Source: CAD feature listing. Evaluate the final solid. Frame: model axes, mm. Face numbers are marked on the shaded views. A direction names the side the tool comes from. Give positions to 0.01 mm unless a question says otherwise; leave off trailing zeros. Write each loop counter-clockwise with the first axis right and the second up, starting at its lowest first coordinate (ties: lowest second). Pieces come first, ordered by that corner, then holes.
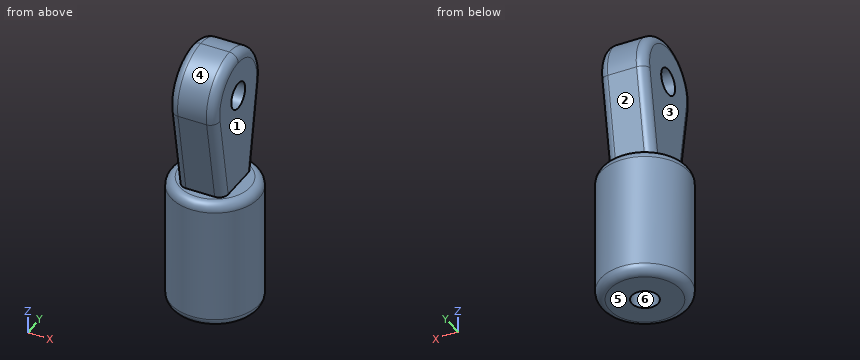
Autodesk Inventor part; units mm, degrees
ref_plane "YZ Plane" through (0, 0, 0) normal (1, 0, 0) x (0, 1, 0)
ref_plane "XZ Plane" through (0, 0, 0) normal (0, 1, 0) x (-1, 0, 0)
ref_plane "XY Plane" through (0, 0, 0) normal (0, 0, 1) x (1, 0, 0)
sketch "Boceto1" plane through (0, 0, 0) normal (0, 0, 1) x (1, 0, 0)
  circle A0 centre (0, 0) radius 10
  dimension "d0" = 20
extrude "Extrusión1" add sketch "Boceto1" along normal blind 30
sketch "Boceto2" plane through (0, 0, 0) normal (1, 0, 0) x (0, 1, 0)
  line L0 (10, 30) -> (-10, 30)
  line L1 (-10, 0) -> (10, 0)
  line L2 (10, 30) -> (-10, 30)
  line L3 (6.3751, 30) -> (9.8481, 49.6962)
  arc A0 (9.8481, 49.6962) -> (0, 61.4326) centre (0, 51.4326) ccw
  line L4 (0, 73.9906) -> (0, 23.9809)
  line L5 (-6.3751, 30) -> (-9.8481, 49.6962)
  arc A1 (0, 61.4326) -> (-9.8481, 49.6962) centre (0, 51.4326) ccw
  line L6 (6.3751, 30) -> (-6.3751, 30)
  point P0 (0, 0)
  point P1 (0, 30)
  dimension "d3" = 10
  dimension "d4" = 20
  dimension "d5" = 100
extrude "Extrusión2" add sketch "Boceto2" along normal mid plane 10.5
hole "Agujero1" at (5.25, 0, 51.4326) direction (-1, 0, 0) diameter 6 end through all
hole "Agujero2" at (0, 0, 0) direction (0, 0, 1) diameter 6 depth 26 tip angle 118
fillet "Empalme1" radius 2 8 edges at (5.25, -8.1116, 39.8481) (5.25, 8.1116, 39.8481) (5.25, -7.6604, 57.8605) (-5.25, 8.1116, 39.8481) (-5.25, -8.1116, 39.8481) (-5.25, 7.6604, 57.8605) (-10, 0, 30) (-10, 0, 0)
properties part number "wheel_shock_end"
1. Mould query, pull axis Y, two halves, no side actions, for the marked faces 4, 5 and 6. Classes: +Y half, -Y half, draft (parallel to the pull), parting line (faces both ways), or undercut.
2. Line query: L1, parallel to Y at x = 0, z = 12.75; L2, parallel to Z at x = -6, y = 3.5; L3, parallel to X at y = -4, z = 45. Output: solid intervals per line, ascending.
3. Cut plane A-A, the plane z = 16. Return the cut outline in (x, y).
4. Access query for the marked faces 1, 2 and 3. Directions: +Z, -Z, +X, -X, +Y, -Y. A direction counts if a zero-diameter tool reaches every point of the face in a straight line with its end or side. Return the directions, or none.
5. Contact query for flat-ended pins moving along their axis: P1, Ø4, axis at x = 3.5, z = 28.5, coming from the -Y side; P2, Ø3, axis at y = 6.5, z = 50, coming from the -X side; P3, Ø12, axis at x = 1.5, y = 1.5, coming from the -Z side; P4, Ø2, axis at x = 3.5, y = 2, coming from the +Z side. Output: stop coordinate, or through.
Response values:
1. face 4: -Y half
1. face 5: draft
1. face 6: undercut
2. L1: y = -10 to -3, 3 to 10
2. L2: z = 0 to 30
2. L3: x = -5.25 to 5.25
3. outline: circle Ø20 at (0, 0); hole circle Ø6 at (0, 0)
4. face 1: +Z, +X, +Y, -Y
4. face 2: +X, -X, +Y
4. face 3: +Z, -X, +Y, -Y
5. P1: stops at y = -9.88
5. P2: stops at x = -5.25
5. P3: stops at z = 0
5. P4: stops at z = 61.38
